Part model, mm, in its own coordinate system. A direction names the side the tool comes from. Coordinates: 2 decimals unless noted, no trailing zeros. Write each loop counter-clockwise with the first axis right and the second up, starting at its lowest first coordinate (ties: lowest second). Pieces come first, ordered by that corner, then holes. Notation, with made-up numbers: (70.25, 15.5) -> (114.25, 15.5) arc R25 cw to (114.25, 40.5) -> close; hole circle Ø11 at (2.5, -10.75). An arc over 180 degrees is marked (long way). Write item = value, one per line.
from build123d import *

# Parameters (mm, degrees)
SKETCH1_R           = 4.2
BOSS_EXTRUDE1_DEPTH = 10


with BuildPart() as part:
    # Sketch1 → Boss-Extrude1 (new body)
    with BuildSketch(Plane(origin=(0, 0, 0), x_dir=(1, 0, 0), z_dir=(0, 1, 0))):
        with BuildLine():
            Line((133, 24), (133, 21))
            Line((133, 21), (173, 21))
            Line((173, 21), (181, 21))
            Line((181, 21), (181, 24))
            Line((181, 24), (173, 24))
            Line((173, 24), (161.223447426, 24))
            ThreePointArc((161.223447426, 24), (154.671414284, 51.436889518), (143.48714405, 77.333301316))
            ThreePointArc((143.48714405, 77.333301316), (142.822320311, 78.554343107), (142.147106039, 79.769669954))
            ThreePointArc((142.147106039, 79.769669954), (126.959135765, 82.689852197), (123.107582845, 67.710952187))
            ThreePointArc((123.107582845, 67.710952187), (132.585040112, 46.491473825), (138.435002799, 24))
            Line((138.435002799, 24), (133, 24))
        make_face()
        with Locations(Location((148.576085497, 31.070096853, 0), (0, 0, 270))):
            Circle(SKETCH1_R, mode=Mode.SUBTRACT)
        with Locations(Location((144.782134175, 45.588789451, 0), (0, 0, 270))):
            Circle(SKETCH1_R, mode=Mode.SUBTRACT)
        with Locations(Location((139.573135396, 59.661913947, 0), (0, 0, 270))):
            Circle(SKETCH1_R, mode=Mode.SUBTRACT)
        with BuildLine():
            ThreePointArc((129.319915673, 71.127825148), (130.975900362, 76.832009114), (136.680084327, 75.176024425))
            ThreePointArc((136.680084327, 75.176024425), (137.067945069, 74.19682809), (137.2, 73.151924787))
            ThreePointArc((137.2, 73.151924787), (134.044903303, 69.083979717), (129.319915673, 71.127825148))
        make_face(mode=Mode.SUBTRACT)
    extrude(amount=BOSS_EXTRUDE1_DEPTH)


solid = part.part
Q1. Saw through at D-D on x = 167. Give the cut face in (y, z), and give its area (3 significant figures).
Model answer:
outline = (0, -24) -> (10, -24) -> (10, -21) -> (0, -21) -> close
area = 30.0 mm²
Q2. Saw through at C-C on y = 3.25. Give the cut face in (x, z) (3 decimals).
Model answer:
outline = (123.108, -67.711) arc R11.29 ccw to (142.147, -79.77) arc R163 ccw to (143.487, -77.333) arc R163 ccw to (161.223, -24) -> (181, -24) -> (181, -21) -> (133, -21) -> (133, -24) -> (138.435, -24) arc R140.5 cw to start; hole circle Ø8.4 at (133, -73.152); hole circle Ø8.4 at (139.573, -59.662); hole circle Ø8.4 at (144.782, -45.589); hole circle Ø8.4 at (148.576, -31.07)
Q3. Mould opens along X. For faces 4 (the face through (181, 5, -22)), 5 (the face through (137.018, 4.93, -62.995)), 6 (the face through (142, 10, -53)) say: released by +X, released by -X, zero draft, split by the parting line, or undercut.
Model answer:
face_4 = released by +X
face_5 = undercut
face_6 = zero draft
Q4. Saw through at B-B on x = 150. Give the cut face in (y, z), and give its area (3 significant figures).
Model answer:
outline = (0, -63.79) -> (10, -63.79) -> (10, -35.02) -> (0, -35.02) -> close; (0, -27.12) -> (10, -27.12) -> (10, -21) -> (0, -21) -> close
area = 349 mm²
Q5. Probe line 1 (Z direction, x = 142, y = 5); line 2 (Z direction, x = 139, y = 1.25); line 3 (Z direction, x = 142.5, y = 6.75). List the from-to ranges inside material, lowest first. Write a range as from..to.
Model answer:
line_1 = -79.97..-63.09, -56.23..-48.74, -42.44..-21
line_2 = -82.72..-63.82, -55.5..-21
line_3 = -79.14..-62.67, -56.65..-49.11, -42.06..-21
Q6. Which spindle directions (+Z, -Z, +X, -X, +Y, -Y) get a long thin tool onto all of the face, cutting with end or side? Do faces 1 (the face through (132.477, 4.93, -46.799)), 2 (the face through (171, 5, -24)), 3 (the face through (133, 5, -23)). Say none if no direction does.
Model answer:
face_1 = -X, +Y, -Y
face_2 = -Z, +X, +Y, -Y
face_3 = +Z, -X, +Y, -Y
Q7. Saw through at A-A on z = -48. Give the cut face in (x, y).
Model answer:
outline = (132.05, 0) -> (141.34, 0) -> (141.34, 10) -> (132.05, 10) -> close; (148.22, 0) -> (155.77, 0) -> (155.77, 10) -> (148.22, 10) -> close
Q8. Pin check, flat tips, straight feed: pin 1 (6 mm diameter, centred on y = 7.5, z = -54, fed in from +X); pin 2 (1.5 mm diameter, centred on y = 3, z = -23, fed in from -X); pin 3 (2 mm diameter, centred on y = 7, z = -47, fed in from -X). Stop position of each tip, or through.
Model answer:
pin_1 = 154.82
pin_2 = 133
pin_3 = 132.05
